Autodesk Inventor part; units mm, degrees
ref_plane "YZ Plane" through (0, 0, 0) normal (1, 0, 0) x (0, 1, 0)
ref_plane "XZ Plane" through (0, 0, 0) normal (0, 1, 0) x (-1, 0, 0)
ref_plane "XY Plane" through (0, 0, 0) normal (0, 0, 1) x (1, 0, 0)
sketch "Sketch2" plane through (0, 0, 0) normal (0, 1, 0) x (-1, 0, 0)
  line L0 (15, 20.15) -> (20.15, 15)
  line L1 (20.15, 15) -> (20.15, -15)
  line L2 (20.15, -15) -> (15, -20.15)
  line L3 (15, -20.15) -> (-15, -20.15)
  line L4 (-15, -20.15) -> (-20.15, -15)
  line L5 (-20.15, -15) -> (-20.15, 15)
  line L6 (-20.15, 15) -> (-15, 20.15)
  line L7 (-15, 20.15) -> (15, 20.15)
  point P0 (0, 0)
  point P1 (20.15, 0)
  point P2 (0, -20.15)
  dimension "d2" = 30
  dimension "d3" = 40.3
  dimension "d4" = 135
extrude "Extrusion1" add sketch "Sketch2" along normal mid plane 34
sketch "Sketch7" plane through (0, 17, 0) normal (0, 1, 0) x (1, 0, 0)
  circle A0 centre (0, 0) radius 11
  dimension "d27" = 22
extrude "Extrusion3" add sketch "Sketch7" along normal blind 2
sketch "Sketch8" plane through (0, 19, 0) normal (0, 1, 0) x (1, 0, 0)
  circle A0 centre (0, 0) radius 4
  dimension "d30" = 8
extrude "Extrusion4" cut sketch "Sketch8" against normal blind 1
sketch "Sketch9" plane through (0, 18, 0) normal (0, 1, 0) x (1, 0, 0)
  circle A0 centre (0, 0) radius 2.5
  dimension "d33" = 5
extrude "Extrusion5" add sketch "Sketch9" along normal blind 23
sketch "Sketch10" plane through (-15, 17, 20.15) normal (0, 0, 1) x (1, 0, 0)
  line L0 (30, 0) -> (30, -34)
  line L1 (0, 0) -> (30, 0)
  line L2 (0, -34) -> (0, 0)
  line L3 (30, -34) -> (0, -34)
  line L4 (0, 0) -> (30, 0)
  line L5 (30, 0) -> (30, -10)
  line L6 (30, -10) -> (0, -10)
  line L7 (0, -10) -> (0, 0)
  line L8 (0, 0) -> (30, -10) construction
  line L9 (30, 0) -> (0, -10) construction
  line L10 (0, -24) -> (30, -24)
  line L11 (30, -24) -> (30, -34)
  line L12 (30, -34) -> (0, -34)
  line L13 (0, -34) -> (0, -24)
  line L14 (0, -24) -> (30, -34) construction
  line L15 (30, -24) -> (0, -34) construction
  line L16 (0, 0) -> (30, 0)
  point P0 (15, -17)
  point P1 (15, -5)
  point P2 (15, -29)
  dimension "d36" = 10
  dimension "d37" = 10
extrude "Extrusion6" add sketch "Sketch10" along normal blind 1 contours L0 L6 L2 L1 | L0 L3 L2 L10
mirror "Mirror1" about plane through (0, 0, 0) normal (0, 0, 1) of "Extrusion6"
sketch "Sketch11" plane through (20.15, -17, -15) normal (1, 0, 0) x (0, 0, -1)
  line L0 (0, 34) -> (0, 0)
  line L1 (-30, 34) -> (0, 34)
  line L2 (-30, 34) -> (-30, 0)
  line L3 (0, 0) -> (-30, 0)
  line L4 (-30, 34) -> (0, 34)
  line L5 (0, 34) -> (0, 24)
  line L6 (0, 24) -> (-30, 24)
  line L7 (-30, 24) -> (-30, 34)
  line L8 (-30, 34) -> (0, 24) construction
  line L9 (0, 34) -> (-30, 24) construction
  line L10 (-30, 10) -> (0, 10)
  line L11 (0, 10) -> (0, 0)
  line L12 (0, 0) -> (-30, 0)
  line L13 (-30, 0) -> (-30, 10)
  line L14 (-30, 10) -> (0, 0) construction
  line L15 (0, 10) -> (-30, 0) construction
  line L16 (-30, 34) -> (0, 34)
  point P0 (-15, 17)
  point P1 (-15, 29)
  point P2 (-15, 5)
  dimension "d40" = 10
extrude "Extrusion7" add sketch "Sketch11" along normal blind 1 contours L0 L6 L2 L1 | L0 L3 L2 L10
mirror "Mirror2" about plane through (0, 0, 0) normal (1, 0, 0) of "Extrusion7"
sketch "Sketch12" plane through (-15, -7, 20.15) normal (-0.7071, 0, 0.7071) x (0.7071, 0, 0.7071)
  line L0 (0, -10) -> (0, 0)
  line L1 (0, 0) -> (0, 14)
  line L2 (0, 14) -> (0, 24)
  line L3 (-7.2832, 24) -> (0, 24)
  line L4 (-7.2832, 24) -> (-7.2832, 14)
  line L5 (-7.2832, 14) -> (-7.2832, 0)
  line L6 (-7.2832, 0) -> (-7.2832, -10)
  line L7 (0, -10) -> (-7.2832, -10)
  line L8 (-7.2832, 24) -> (0, 24)
  line L9 (0, 24) -> (0, 14)
  line L10 (0, 14) -> (-7.2832, 14)
  line L11 (-7.2832, 14) -> (-7.2832, 24)
  line L12 (-7.2832, 24) -> (0, 14) construction
  line L13 (0, 24) -> (-7.2832, 14) construction
  line L14 (-7.2832, 0) -> (0, 0)
  line L15 (0, 0) -> (0, -10)
  line L16 (0, -10) -> (-7.2832, -10)
  line L17 (-7.2832, -10) -> (-7.2832, 0)
  line L18 (-7.2832, 0) -> (0, -10) construction
  line L19 (0, 0) -> (-7.2832, -10) construction
  line L20 (-7.2832, 24) -> (0, 24)
  line L21 (0, -10) -> (-7.2832, -10)
  point P0 (-3.6416, 7)
  point P1 (-3.6416, 19)
  point P2 (-3.6416, -5)
  dimension "d43" = 10
  dimension "d44" = 10
extrude "Extrusion8" add sketch "Sketch12" along normal blind 1 contours L7 L6 L14 L0 | L10 L4 L3 L2
sketch "Sketch14" plane through (-15, 7, 21.15) normal (-1, 0, 0) x (0, 0, 1)
  line L0 (-1, 0) -> (-1, 10)
  line L1 (-1, 0) -> (0, 0)
  line L2 (0, 10) -> (0, 0)
  line L3 (-1, 10) -> (0, 10)
  line L4 (-1, -24) -> (-1, -14)
  line L5 (-1, -24) -> (0, -24)
  line L6 (0, -14) -> (0, -24)
  line L7 (-1, -14) -> (0, -14)
  point P0 (-21.15, -7)
extrude "Extrusion9" add sketch "Sketch14" along normal up to surface surface through (-18.2821, -12, 18.2821) normal (-0.7071, 0, 0.7071)
sketch "Sketch15" plane through (-21.15, 7, 15) normal (0, 0, 1) x (1, 0, 0)
  line L0 (1, 10) -> (1, 0)
  line L1 (1, 10) -> (0, 10)
  line L2 (0, 10) -> (0, 0)
  line L3 (1, 0) -> (0, 0)
  line L4 (1, -14) -> (1, -24)
  line L5 (1, -14) -> (0, -14)
  line L6 (0, -14) -> (0, -24)
  line L7 (1, -24) -> (0, -24)
  point P0 (21.15, -7)
extrude "Extrusion10" add sketch "Sketch15" along normal up to surface surface through (-18.2821, -12, 18.2821) normal (-0.7071, 0, 0.7071)
mirror "Mirror3" about plane through (0, 0, 0) normal (1, 0, 0) of "Extrusion8", "Extrusion9", "Extrusion10"
mirror "Mirror4" about plane through (0, 0, 0) normal (0, 0, 1) of "Extrusion8", "Extrusion9", "Extrusion10", "Mirror3"
sketch "Sketch17" plane through (0, 17, 0) normal (0, 1, 0) x (1, 0, 0)
  line L0 (-21.15, -15.4142) -> (-15.4142, -21.15)
  line L1 (-15.4142, -21.15) -> (15.4142, -21.15)
  line L2 (21.15, -15.4142) -> (15.4142, -21.15)
  line L3 (21.15, -15.4142) -> (21.15, 15.4142)
  line L4 (21.15, 15.4142) -> (15.4142, 21.15)
  line L5 (15.4142, 21.15) -> (-15.4142, 21.15)
  line L6 (-21.15, 15.4142) -> (-15.4142, 21.15)
  line L7 (-21.15, 15.4142) -> (-21.15, -15.4142)
  circle A0 centre (0, 0) radius 11
  circle A1 centre (-15.5, -15.5) radius 1.5
  circle A2 centre (-15.5, 15.5) radius 1.5
  circle A3 centre (15.5, 15.5) radius 1.5
  circle A4 centre (15.5, -15.5) radius 1.5
  dimension "d53" = 3
  dimension "d54" = 31
  dimension "d55" = 31
  dimension "d57" = 15.5
  dimension "d66" = 15.5
hole "Hole3" at (-15.5, 17, 15.5) at (-15.5, 17, -15.5) at (15.5, 17, -15.5) at (15.5, 17, 15.5) direction (0, -1, 0) diameter 3 depth 4.5
sketch "Sketch19" plane through (0, 41, 0) normal (0, 1, 0) x (1, 0, 0)
  circle A0 centre (0, 0) radius 2.5
  circle A1 centre (0, 0) radius 2.5
  line L0 (-1.5, -2) -> (1.5, -2)
  dimension "d69" = 4.5
extrude "Extrusion12" cut sketch "Sketch19" against normal blind 15 contours L0 A0 picked at (-0.3466, -2.0912)
ref_plane "Work Plane1" through (0, 0, 0) normal (1, 0, 0) x (0, 1, 0)
ref_plane "Work Plane2" through (0, 0, 0) normal (-1, 0, 0) x (0, 1, 0)
ref_plane "Work Plane3" through (0, 0, 0) normal (-1, 0, 0) x (0, 1, 0)
properties part number "Motor_paso"
Model file for the job. Use its own axes, mm. A direction names the side the tool comes from. Coordinates: 2 decimals unless noted, no trailing zeros. Write each loop counter-clockwise with the first axis right and the second up, starting at its lowest first coordinate (ties: lowest second). Pieces come first, ordered by that corner, then holes. Notation, with made-up numbers: (-19.75, -35.75) - (-9.75, -35.75) arc R20 ccw to (-9.75, -17.75) - close; hole circle Ø11 at (-23, 57.5). An arc over 180 degrees is marked (long way). Use a Markdown table: item, result. Add a question column.
Item 1: 3-axis set-ups, long thin cutter, end or side, ignore diameter. For faces 1 (the face through (20.15, 0, 0)), 2 (the face through (-15.57, 14.72, -17)), 3 (the face through (-20.15, 0, 0)): which of +Z, -Z, +X, -X, +Y, -Y reach the whole face in a straight line?
Item 2: Band-saw the part on C-C, the plane x = 0. Write the cut outline in (y, z).
Item 3: Band-saw the part on D-D, the plane y = -12. Write the cut outline in (x, z).
Item 4: Band-saw the part on A-A, the plane z = 0. Write the cut outline in (x, y), and give its area (3 significant figures).
Item 5: Drop flat-ended pins along their axis: pin 1 (8 mm diameter, centred on x = -3, y = 29, fed in from -Z); pin 2 (1.5 mm diameter, centred on x = 7, z = -13.5, fed in from +Y); pin 3 (2 mm diameter, centred on y = -2.5, z = 7.5, fed in from -X). Give the stop position or say it passes through.
Item 6: Drill centre lines: line 1 along X through (y, z) = (13.5, 15.5); line 2 along Z through (x, y) = (5, -4.5); line 3 along Y through (x, z) = (-3, -15). Where is each one in solid material? Low to high.
Item 7: Band-saw the part on B-B, the plane y = -5. Write the cut outline in (x, z), and give its area (3 significant figures).
Item 8: Two-plate mould, pull along Y, no slides. Class faces 4 (the face through (0, 0, 20.15)), 5 (the face through (-15.57, 14.72, 14)), 6 (the face through (0, 41, 0)): pulls with the +Y half, pulls with the -Y half, needs draft (parallel to the pull), parting line crosses it, or undercut.
A:
| question | item | result |
|---|---|---|
| 1 | face 1 | +Z, -Z, +X |
| 1 | face 2 | +Y |
| 1 | face 3 | +Z, -Z, -X |
| 2 | outline | (-17, -21.15) - (-7, -21.15) - (-7, -20.15) - (7, -20.15) - (7, -21.15) - (17, -21.15) - (17, -11) - (19, -11) - (19, -4) - (18, -4) - (18, -2.5) - (41, -2.5) - (41, 2) - (26, 2) - (26, 2.5) - (18, 2.5) - (18, 4) - (19, 4) - (19, 11) - (17, 11) - (17, 21.15) - (7, 21.15) - (7, 20.15) - (-7, 20.15) - (-7, 21.15) - (-17, 21.15) - close |
| 3 | outline | (-21.15, -15.41) - (-15.41, -21.15) - (15.41, -21.15) - (21.15, -15.41) - (21.15, 15.41) - (15.41, 21.15) - (-15.41, 21.15) - (-21.15, 15.41) - close |
| 4 | outline | (-21.15, -17) - (21.15, -17) - (21.15, -7) - (20.15, -7) - (20.15, 7) - (21.15, 7) - (21.15, 17) - (11, 17) - (11, 19) - (4, 19) - (4, 18) - (2.5, 18) - (2.5, 41) - (-2.5, 41) - (-2.5, 18) - (-4, 18) - (-4, 19) - (-11, 19) - (-11, 17) - (-21.15, 17) - (-21.15, 7) - (-20.15, 7) - (-20.15, -7) - (-21.15, -7) - close |
| 4 | area | 1,560 mm² |
| 5 | pin 1 | stops at z = -2.5 |
| 5 | pin 2 | stops at y = 17 |
| 5 | pin 3 | stops at x = -20.15 |
| 6 | line 1 | x = -21.06 to -17, -14 to 14, 17 to 21.06 |
| 6 | line 2 | z = -20.15 to 20.15 |
| 6 | line 3 | y = -17 to 17 |
| 7 | outline | (-20.15, -15) - (-15, -20.15) - (15, -20.15) - (20.15, -15) - (20.15, 15) - (15, 20.15) - (-15, 20.15) - (-20.15, 15) - close |
| 7 | area | 1,570 mm² |
| 8 | face 4 | undercut |
| 8 | face 5 | needs draft |
| 8 | face 6 | pulls with the +Y half |
